Geometry: final body of the model. Coordinates: model frame, mm. Face numbers are marked on the shaded views. A direction names the side the tool comes from. Give positions to 0.01 mm unless a question says otherwise; leave off trailing zeros. Loops run counter-clockwise (first coordinate to the right, second up) from the corner with the lowest first, then second, coordinate; pieces in that order, holes last.
1. Section B-B, the plane y = -38.5. Output: boundary loops of the cut face in (x, z), then the cut area to 3 significant figures.
2. Material intervals for line 1 along Y through (x, z) = (-4.5, -29); line 2 along Z through (x, y) = (2, -20.4) (3 decimals); line 3 along Z through (x, y) = (4.25, -28), sorted ascending.
3. Draft query along Y for the marked faces 1, 2 and 3. Return one class per face: +Y half, -Y half, draft (parallel to the pull), parting line (faces both ways), or undercut.
4. Section A-A, the plane y = -30. Output: boundary loops of the cut face in (x, z) (3 decimals), then the cut area to 3 significant figures.
5. Section C-C, the plane z = -33. Output: boundary loops of the cut face in (x, y), then the cut area to 3 significant figures.
6. Section D-D, the plane x = 2. State how many separate pieces and enclosed holes the cut face has, then the cut area to 3 significant figures.
7. Access query for the marked faces 4 and 5. Directions: +Z, -Z, +X, -X, +Y, -Y. A direction counts if a zero-diameter tool reaches every point of the face in a straight line with its end or side. Return the directions, or none.
8. First-contact query: P1, Ø5, axis at x = 10, y = -25.5, coming from the +Z side; P2, Ø4, axis at x = 6, z = -28, coming from the -Y side; P3, Ø3, axis at x = 1, z = -20, coming from the +Y side. Flat tips, straight axial feed; report the tip coordinate or a pass-through.
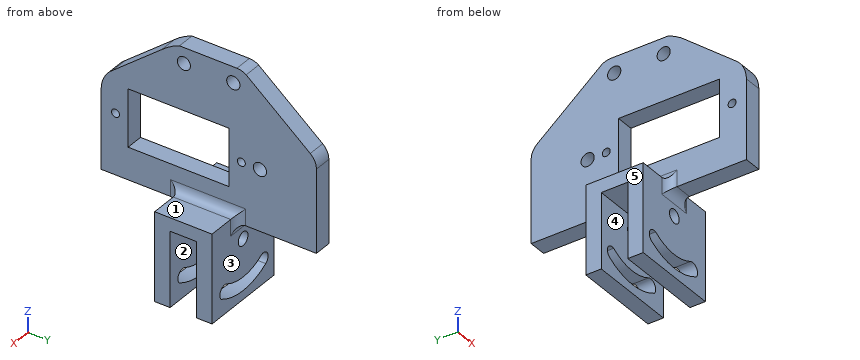
Autodesk Inventor part; units mm, degrees
ref_plane "YZ Plane" through (0, 0, 0) normal (1, 0, 0) x (0, 1, 0)
ref_plane "XZ Plane" through (0, 0, 0) normal (0, 1, 0) x (-1, 0, 0)
ref_plane "XY Plane" through (0, 0, 0) normal (0, 0, 1) x (1, 0, 0)
sketch "Szkic1" plane through (0, 0, 0) normal (1, 0, 0) x (0, 1, 0)
  line L0 (0, 1.0111) -> (0, -17.7395)
  line L1 (0, -17.7395) -> (-48.7346, -17.7395)
  line L2 (-48.7346, -17.7395) -> (-48.7346, 0.2105)
  arc A0 (-46.1212, 5.2996) -> (-48.7346, 0.2105) centre (-42.4729, 0.2105) ccw
  line L3 (-46.1212, 5.2996) -> (-35.0263, 14.1821)
  arc A1 (-31.0007, 16.5663) -> (-35.0263, 14.1821) centre (-26.6278, 4.5922) ccw
  arc A2 (-15.4691, 15.5487) -> (-18, 16.5663) centre (-18, 12.9101) ccw
  arc A3 (0, 1.0111) -> (-1.3971, 3.9699) centre (-3.8316, 1.0111) ccw
  line L4 (-15.8982, 15.9018) -> (-1.3971, 3.9699)
  line L5 (-18, 16.5663) -> (-31.0007, 16.5663)
  circle A4 centre (-18.8067, 13.002) radius 1.5007
  circle A5 centre (-30, 13.0039) radius 1.4888
  circle A6 centre (-45.4922, -4) radius 0.9
  circle A7 centre (-12.7873, -3.975) radius 1.5
  circle A8 centre (-16.9979, -3.975) radius 0.9
  line L6 (-19.7721, 2.5223) -> (-19.7721, -10.4698)
  line L7 (-19.7721, -10.4698) -> (-42.6386, -10.4698)
  line L8 (-42.6386, -10.4698) -> (-42.6386, 2.5223)
  line L9 (-42.6386, 2.5223) -> (-19.7721, 2.5223)
  point P0 (0, 0)
  point P1 (0, -22.6354)
  dimension "d0" = 1.8
  dimension "d1" = 3
  dimension "d2" = 1.8
extrude "Wyciągnięcie proste1" add sketch "Szkic1" along normal blind 4 contours L0 L1 L2 A0 L3 A1 L5 A2 L4 A3
sketch "Szkic2" plane through (4, 0, 0) normal (1, 0, 0) x (0, 0, -1)
  line L0 (-16.5663, -18) -> (-16.5663, -31.0007)
  line L1 (-16.5663, -24.5004) -> (42, -24.5004)
  line L2 (16, -18.0004) -> (36, -18.0004)
  line L3 (36, -18.0004) -> (36, -31.0004)
  line L4 (36, -31.0004) -> (16, -31.0004)
  line L5 (16, -31.0004) -> (16, -18.0004)
  point P0 (0, 0)
  dimension "d5" = 20
  dimension "d6" = 13
extrude "Wyciągnięcie proste2" add sketch "Szkic2" against normal blind 12
sketch "Szkic3" plane through (-8, 0, 0) normal (-1, 0, 0) x (0, 0, 1)
  line L0 (-17.7395, -18.0004) -> (-16, -18.0004)
  line L1 (-36, -31.0004) -> (-17.7395, -31.0004)
  line L2 (-16, -18.0004) -> (-36, -18.0004)
  line L3 (-36, -18.0004) -> (-36, -31.0004)
  line L4 (-36, -31.0004) -> (-16, -31.0004)
  line L5 (-16, -31.0004) -> (-16, -18.0004)
  point P0 (0, 0)
extrude "Wyciągnięcie proste3" add sketch "Szkic3" against normal blind 20
sketch "Szkic4" plane through (-8, -31.0004, -36) normal (0, 0, -1) x (-1, 0, 0)
  point P0 (-8, 31.0004)
sketch "Szkic5" plane through (-8, 0, 0) normal (-1, 0, 0) x (0, 0, 1)
  line L0 (-36, -18.0004) -> (-36, -31.0004)
  line L1 (-36, -27.5004) -> (-19, -27.5004)
  line L2 (-19, -27.5004) -> (-19, -21.5004)
  line L3 (-19, -21.5004) -> (-36, -21.5004)
  line L4 (-36, -21.5004) -> (-36, -27.5004)
  line L5 (-16, -31.0004) -> (-16, -18.0004)
  line L6 (-16, -24.5004) -> (-39.2975, -24.5004)
  line L7 (-20, -27) -> (-36, -27)
  line L8 (-36, -27) -> (-36, -21)
  line L9 (-36, -21) -> (-20, -21)
  line L10 (-20, -21) -> (-20, -27)
  point P0 (0, 0)
  dimension "d23" = 6
fillet "Zaokrąglenie1" radius 2 8 edges at (0, -31.0004, -16.8697) (0, -24.5004, -16) (0, -18.0004, -16.8697) (2, -18.0004, -17.7395) (4, -18.0004, -16.8697) (4, -24.5004, -16) (4, -31.0004, -16.8697) (2, -31.0004, -17.7395)
sketch "Szkic6" plane through (-8, -18.0004, -16) normal (0, 1, 0) x (1, 0, 0)
  line L0 (20, 20) -> (0, 20)
  line L1 (10, 20) -> (10, -8)
  circle A0 centre (10, 6.4693) radius 1.55
  arc A1 (15.9953, 14.4545) -> (4.2067, 14.6022) centre (10, 6.4693) ccw
  arc A2 (17.6193, 17.0025) -> (1.6495, 16.4327) centre (10, 6.4693) ccw
  arc A3 (15.9953, 14.4545) -> (17.6193, 17.0025) centre (16.7323, 15.7763) ccw
  arc A4 (1.6495, 16.4327) -> (4.2067, 14.6022) centre (3.2422, 15.9562) ccw
  line L2 (15.8971, 14.5272) -> (16.0005, 14.4516)
  line L3 (1.7865, 16.546) -> (1.6196, 16.3179)
  point P0 (8, -16)
  dimension "d14" = 3.1
  dimension "d17" = 26
extrude "Wyciągnięcie proste5" cut sketch "Szkic6" against normal blind 20 contours A0 L1 | L1 A0
sketch "Szkic7" plane through (-8, -18.0004, -16) normal (0, 1, 0) x (1, 0, 0)
  line L0 (0, 20) -> (20, 20)
  line L1 (10, 20) -> (10, -4.2283)
  line L2 (20, 20) -> (20, 0)
  circle A0 centre (10, 4) radius 11
  circle A1 centre (10, 4) radius 14.025
  arc A2 (15.2148, 13.6853) -> (17.0707, 16.1122) centre (15.9483, 15.0475) ccw
  arc A3 (2.7167, 15.9856) -> (3.9993, 13.2191) centre (3.5134, 14.6744) ccw
  point P0 (8, -16)
  dimension "d18" = 10
  dimension "d19" = 22
  dimension "d20" = 28.05
extrude "Wyciągnięcie proste6" cut sketch "Szkic7" against normal blind 20 contours A1 A2 A0 L1 | L1 A0 A3 A1
extrude "Wyciągnięcie proste7" cut sketch "Szkic5" against normal up to next contours L3 L10 L6 L0 | L6 L10 L7 L0 | L3 L2 L6 L10 | L7 L10 L6 L2 L1 L0
properties part number "czesc glowna chwytaka"
Answers below:
1. outline: (0, -17.74) - (4, -17.74) - (4, -10.47) - (0, -10.47) - close; (0, 2.52) - (4, 2.52) - (4, 11.4) - (0, 11.4) - close
1. area: 64.6 mm2
2. line 1: y = -31 to -27.5, -21.5 to -18
2. line 2: z = -36 to -34.025, -31 to -24.019, -20.919 to -10.47, 2.522 to 16.566
2. line 3: z = -36 to -33.84, -30.77 to -14.97
3. face 1: draft
3. face 2: undercut
3. face 3: +Y half
4. outline: (-8, -36) - (12, -36) - (12, -16) - (6, -16) arc R2 cw to (4, -14) - (4, -10.47) - (0, -10.47) - (0, -14) arc R2 cw to (-2, -16) - (-8, -16) - close; (0, 2.522) - (4, 2.522) - (4, 11.515) - (0, 11.515) - close; (0, 14.493) - (4, 14.493) - (4, 16.566) - (0, 16.566) - close; hole (-5.283, -31.986) arc R14.025 ccw to (9.071, -32.112) arc R1.547 ccw to (7.215, -29.685) arc R11 cw to (-4.001, -29.219) arc R1.534 ccw to start; hole circle Ø3.1 at (2, -22.469)
4. area: 414 mm2
5. outline: (-8, -31) - (-3.26, -31) - (-3.26, -27.5) - (-8, -27.5) - close; (-8, -21.5) - (-3.26, -21.5) - (-3.26, -18) - (-8, -18) - close; (7.26, -31) - (12, -31) - (12, -27.5) - (7.26, -27.5) - close; (7.26, -21.5) - (12, -21.5) - (12, -18) - (7.26, -18) - close
5. area: 66.3 mm2
6. separate pieces: 5
6. enclosed holes: 6
6. area: 1,210 mm2
7. face 4: -Z, +X, -X
7. face 5: +Z, -Z, -X, +Y, -Y
8. P1: stops at z = -16
8. P2: stops at y = -31
8. P3: stops at y = -17.57
